Part model, mm, in its own coordinate system. Face numbers are marked on the shaded views. A direction names the side the tool comes from. Give positions to 0.01 mm unless a question says otherwise; leave off trailing zeros. Order: outer loops, then holes, each group sorted by start corner. A loop starts at its lowest first (then second) coordinate and runs counter-clockwise, first axis right, second up.
1. Which spindle directions (+Z, -Z, +X, -X, +Y, -Y) get a long thin tool onto all of the face, cutting with end or side? Do the marked faces 4, 5 and 6. Say none if no direction does.
2. Mould opens along Z. For the marked faces 1, 2 and 3 say: +Z half, -Z half, draft (parallel to the pull), parting line (faces both ways), or undercut.
3. Drop flat-ended pins along their axis: pin 1 Ø1.2 at (y, z) = (-11, 13) entering from +X; pin 2 Ø7.5 at (x, y) = (-2, -13) entering from +Z; pin 3 Ø2 at (x, y) = (-11, -16) entering from +Z; pin 4 Ø1.5 at (x, y) = (-4.5, -7.5) entering from -Z. Give the stop position or say it passes through.
4. Slice it at D-D on y = -5.25. List the corners of the cut face in (x, z).
5. Slice it at A-A on x = -5.5. List the corners of the cut face in (y, z), and give its area (3 significant figures).
6. Slice it at C-C on z = 9.75. List the corners of the cut face in (x, y), and give its area (3 significant figures).
7. Probe line 1 (X direction, y = -10.75, z = 9.25); line 2 (Y direction, x = -10, z = 10.75); line 3 (Y direction, x = -7.75, z = 8.75). List the from-to ranges inside material, lowest first.
from build123d import *

# Parameters (mm, degrees)
PAD_DEPTH                    = 4
BOX055_W                     = 6
BOX055_H                     = 4
BOX055_DEPTH                 = 5
BOX053_W                     = 16
BOX053_H                     = 5
BOX053_DEPTH                 = 10
BOX052_W                     = 16
BOX052_H                     = 13
BOX052_DEPTH                 = 3
BOX051_W                     = 18
BOX051_H                     = 15
BOX051_DEPTH                 = 4
BOX054_W                     = 8
BOX054_H                     = 12
BOX054_DEPTH                 = 2.8
CHAMFER002_SIZE              = 1
FUSION002030_PLACEMENT_ANGLE = 180


with BuildPart() as pad:
    # Sketch → Pad (new body)
    with BuildSketch(Plane.XZ):
        Polygon((1.974622, -4.079123), (2.485922, -4.884556), (2.927797, -4.039041), (3.431991, -4.84464), (3.877564, -4.005196), (4.398553, -4.963919), (4.968336, -4.033368), (5.532483, -4.976998), (6.067618, -4.016618), (6.588753, -4.85016), (7.050054, -3.982073), (7.468007, -4.900089), (8.054056, -4.079123), (8.054056, -3.693932), (1.974622, -3.693932), align=None)
    extrude(amount=PAD_DEPTH)


with BuildPart() as fusion002029:
    # Box055 → Box055 (new body)
    with BuildSketch(Plane(origin=(2, -4, -4), x_dir=(1, 0, 0), z_dir=(0, 0, 1))):
        with Locations((3, 2)):
            Rectangle(BOX055_W, BOX055_H)
    extrude(amount=BOX055_DEPTH)

    # Fusion002029: union Pad
    add(pad.part)


with BuildPart() as fusion002029_1:
    # Fusion002029 placement: moved
    add(fusion002029.part.moved(Location((8, 9.5, 0))))


with BuildPart() as cubo053:
    # Box053 → Box053 (new body)
    with BuildSketch(Plane(origin=(1, 5, -5), x_dir=(1, 0, 0), z_dir=(0, 0, 1))):
        with Locations((8, 2.5)):
            Rectangle(BOX053_W, BOX053_H)
    extrude(amount=BOX053_DEPTH)


with BuildPart() as cubo052:
    # Box052 → Box052 (new body)
    with BuildSketch(Plane(origin=(1, 1, 1), x_dir=(1, 0, 0), z_dir=(0, 0, 1))):
        with Locations((8, 6.5)):
            Rectangle(BOX052_W, BOX052_H)
    extrude(amount=BOX052_DEPTH)


with BuildPart() as cut074:
    # Box051 → Box051 (new body)
    with BuildSketch(Plane.XY):
        with Locations((9, 7.5)):
            Rectangle(BOX051_W, BOX051_H)
    extrude(amount=BOX051_DEPTH)

    # Cut073: cut Cubo052
    add(cubo052.part, mode=Mode.SUBTRACT)

    # Cut074: cut Cubo053
    add(cubo053.part, mode=Mode.SUBTRACT)


with BuildPart() as fusion002030:
    # Box054 → Box054 (new body)
    with BuildSketch(Plane(origin=(8, 1.5, 1), x_dir=(1, 0, 0), z_dir=(0, 0, 1))):
        with Locations((4, 6)):
            Rectangle(BOX054_W, BOX054_H)
    extrude(amount=BOX054_DEPTH)

    # Chamfer002
    chamfer002_edges = [fusion002030.edges().sort_by_distance(p)[0] for p in [
        (8, 7.5, 3.8),
    ]]
    chamfer(chamfer002_edges, length=CHAMFER002_SIZE)


with BuildPart() as fusion002030_1:
    # Chamfer002 placement: moved
    add(fusion002030.part.moved(Location((1, 0, 0))))

    # Fusion002030: union Fusion002029, Cut074
    add(fusion002029_1.part)
    add(cut074.part)


with BuildPart() as fusion002030_2:
    # Fusion002030 placement: moved
    add(fusion002030_1.part.moved(Location((-14, -3.5, 11.5))).rotate(Axis((-14, -3.5, 11.5), (1, 0, 0)), FUSION002030_PLACEMENT_ANGLE))


solid = fusion002030_2.part
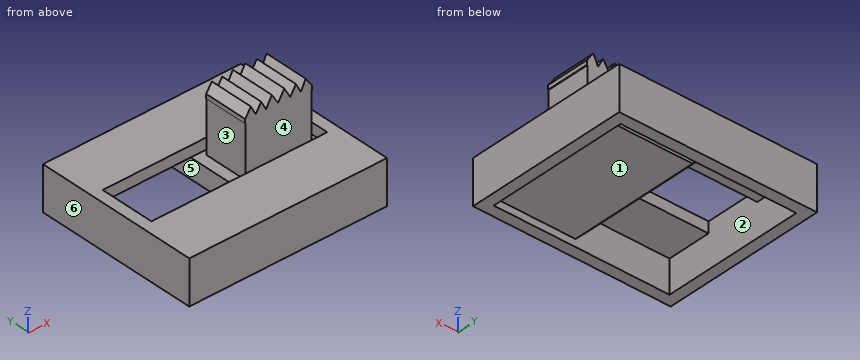
Data:
1. face 4: +Z
1. face 5: -Z
1. face 6: +Z, -Z, -X, +Y, -Y
2. face 1: -Z half
2. face 2: draft
2. face 3: undercut
3. pin 1: stops at x = 2
3. pin 2: stops at z = 16.48
3. pin 3: stops at z = 11.5
3. pin 4: stops at z = 7.7
4. outline: (-14, 7.5) - (-13, 7.5) - (-13, 10.5) - (-5, 10.5) - (-5, 8.7) - (-4, 7.7) - (3, 7.7) - (3, 7.5) - (4, 7.5) - (4, 11.5) - (-14, 11.5) - close
5. outline: (-18.5, 7.5) - (-17.5, 7.5) - (-17.5, 10.5) - (-13.5, 10.5) - (-13.5, 11.5) - (-18.5, 11.5) - close; (-8.5, 10.5) - (-4.5, 10.5) - (-4.5, 7.5) - (-3.5, 7.5) - (-3.5, 11.5) - (-8.5, 11.5) - close
5. area: 16.0 mm2
6. outline: (-14, -18.5) - (4, -18.5) - (4, -3.5) - (-14, -3.5) - close; hole (-13, -17.5) - (3, -17.5) - (3, -17) - (-5, -17) - (-5, -5) - (3, -5) - (3, -4.5) - (-13, -4.5) - close
6. area: 158 mm2
7. line 1: x = -14 to -13, -5 to 4
7. line 2: y = -18.5 to -13.5, -8.5 to -3.5
7. line 3: y = -18.5 to -17.5, -4.5 to -3.5
